Verification items for the finished model (mm, model axes). Face numbers are marked on the shaded views. Coordinates: 2 decimals unless noted, no trailing zeros. Order: outer loops, then holes, each group sorted by start corner. A loop starts at its lowest first (then second) coordinate and runs counter-clockwise, first axis right, second up. Notation, with made-up numbers: (43.25, -34.5) -> (85.25, -34.5) arc R27 ccw to (85.25, -1.5) -> close; hole circle Ø6 at (58, 39.5). An arc over 180 degrees is marked (long way). Use CSV: the item, a comma, the result in double quotes. Start each with the question number.
1) Go/stop test with flat-tipped pins: pin 1 (4 mm diameter, centred on x = 174.5, z = 5.5, fed in from -Y); pin 2 (4 mm diameter, centred on x = 324, y = 81, fed in from -Z); pin 3 (2 mm diameter, centred on x = 390.5, y = 327, fed in from +Z); pin 4 (0.9 mm diameter, centred on x = 370, z = 22, fed in from -Y). Record where each tip stops, or that it passes through.
2) Scan lines: line 1 along X through (y, z) = (389.5, 5); line 2 along Y through (x, z) = (407.5, 6); line 3 along Z through (x, y) = (158.5, 195.5). Record each from-to range of solid material in increasing order.
3) Sectioned sample at C-C on x = 176. Record the boundary of the cut face in (y, z).
4) Sectioned sample at A-A on x = 420. Record the boundary of the cut face in (y, z), then the cut area to 3 significant figures.
5) Release check for a two-part mould opening along X. For the marked faces 1 and 2 record: released by +X, released by -X, zero draft, split by the parting line, or undercut.
6) Sectioned sample at B-B on y = 114.5. Record the boundary of the cut face in (x, z), then the cut area to 3 significant figures.
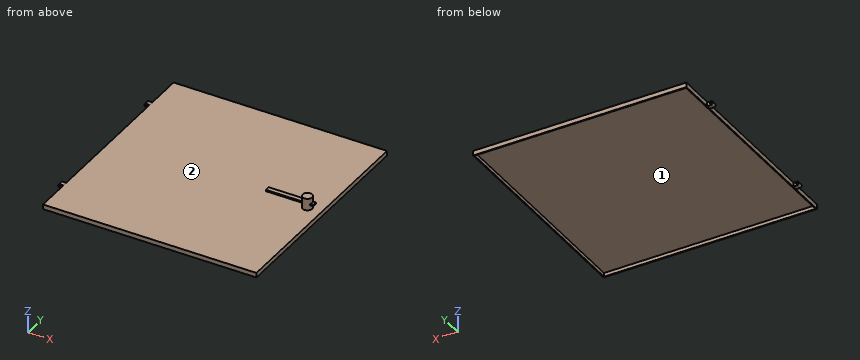
from build123d import *

# Parameters (mm, degrees)
SKETCH1_W           = 450
SKETCH1_H           = 470
BASE_EXTRUDE_DEPTH  = 10
SHELL1_T            = -2
SKETCH2_R           = 2
BOSS_EXTRUDE1_DEPTH = 10
SKETCH3_R           = 10
BOSS_EXTRUDE2_DEPTH = 25
SKETCH4_W           = 100
SKETCH4_H           = 10
BOSS_EXTRUDE3_DEPTH = 3


with BuildPart() as part:
    # Sketch1 → Base-Extrude (new body)
    with BuildSketch(Plane.XY):
        with Locations((225, 235)):
            Rectangle(SKETCH1_W, SKETCH1_H)
    extrude(amount=BASE_EXTRUDE_DEPTH)

    # Shell1
    shell1_openings = [part.faces().sort_by_distance(p)[0] for p in [
        (225, 235, 0),
    ]]
    offset(amount=SHELL1_T, openings=shell1_openings, kind=Kind.INTERSECTION)

    # Sketch2 → Boss-Extrude1 (add)
    with BuildSketch(Plane(origin=(0, 395, 0), x_dir=(-1, 0, 0), z_dir=(0, 1, 0))):
        with BuildLine():
            Line((8, 9), (0, 9))
            Line((0, 9), (0, 1))
            Line((0, 1), (8, 1))
            ThreePointArc((8, 1), (12, 5), (8, 9))
        make_face()
        with Locations(Location((8, 5, 0), (0, 0, 90))):
            Circle(SKETCH2_R, mode=Mode.SUBTRACT)
    boss_extrude1 = extrude(amount=-BOSS_EXTRUDE1_DEPTH)

    # Mirror1: Boss-Extrude1 across plane
    add(boss_extrude1.mirror(Plane.ZX.offset(235)))

    # Sketch3 → Boss-Extrude2 (add)
    with BuildSketch(Plane.XY.offset(10)):
        with Locations(Location((420, 235, 0), (0, 0, 180))):
            Circle(SKETCH3_R)
    extrude(amount=BOSS_EXTRUDE2_DEPTH)

    # Sketch4 → Boss-Extrude3 (add)
    with BuildSketch(Plane.XY.offset(20)):
        with Locations((385, 235)):
            Rectangle(SKETCH4_W, SKETCH4_H)
    extrude(amount=BOSS_EXTRUDE3_DEPTH)


solid = part.part
Answers follow:
1,pin 1,"stops at y = 0"
1,pin 2,"stops at z = 8"
1,pin 3,"stops at z = 10"
1,pin 4,"stops at y = 230"
2,line 1,"x = -12 to -10, -6 to 2, 448 to 450"
2,line 2,"y = 0 to 2, 468 to 470"
2,line 3,"z = 8 to 10"
3,outline,"(0, 0) -> (2, 0) -> (2, 8) -> (468, 8) -> (468, 0) -> (470, 0) -> (470, 10) -> (0, 10) -> close"
4,outline,"(0, 0) -> (2, 0) -> (2, 8) -> (468, 8) -> (468, 0) -> (470, 0) -> (470, 10) -> (245, 10) -> (245, 35) -> (225, 35) -> (225, 10) -> (0, 10) -> close"
4,area,"1,470 mm²"
5,face 1,"undercut"
5,face 2,"zero draft"
6,outline,"(0, 0) -> (2, 0) -> (2, 8) -> (448, 8) -> (448, 0) -> (450, 0) -> (450, 10) -> (0, 10) -> close"
6,area,"932 mm²"
